```python
from build123d import *

# Parameters (mm, degrees)
SKETCH_1_W          = 43
SKETCH_1_H          = 21
EXTRUDE_1_DEPTH     = 1.6
SKETCH_2_R          = 1.5
CUT_EXTRUDE_1_DEPTH = 24.98040867
SKETCH_2_3_R        = 4
EXTRUDE_2_DEPTH     = 10.8
SKETCH_2_4_W        = 12
SKETCH_2_4_H        = 12
EXTRUDE_3_DEPTH     = 7.4
SKETCH_2_5_W        = 10
SKETCH_2_5_H        = 13
EXTRUDE_4_DEPTH     = 4.7
SKETCH_2_6_W        = 9
SKETCH_2_6_H        = 5
EXTRUDE_5_DEPTH     = 10
SKETCH_3_R          = 1.15
EXTRUDE_6_DEPTH     = 1.5


with BuildPart() as part:
    # Sketch 1 → Extrude 1 (new body)
    with BuildSketch(Plane(origin=(0, 0, 0), x_dir=(1, 0, 0), z_dir=(0, 1, 0))):
        Rectangle(SKETCH_1_W, SKETCH_1_H)
    extrude(amount=EXTRUDE_1_DEPTH)

    # Sketch 2 → Cut-Extrude 1 (cut, through all)
    with BuildSketch(Plane(origin=(0, 1.6, 0), x_dir=(1, 0, 0), z_dir=(0, 1, 0))):
        with Locations(Location((-15, 8, 0), (0, 0, 270))):
            Circle(SKETCH_2_R)
        with Locations(Location((15, -8, 0), (0, 0, 270))):
            Circle(SKETCH_2_R)
    extrude(amount=-CUT_EXTRUDE_1_DEPTH, mode=Mode.SUBTRACT)

    # Sketch 2_3 → Extrude 2 (add)
    with BuildSketch(Plane(origin=(0, 1.6, 0), x_dir=(1, 0, 0), z_dir=(0, 1, 0))):
        with Locations(Location((-17.5, 0, 0), (0, 0, 180))):
            Circle(SKETCH_2_3_R)
        with Locations((17.5, 0)):
            Circle(SKETCH_2_3_R)
    extrude(amount=EXTRUDE_2_DEPTH)

    # Sketch 2_4 → Extrude 3 (add)
    with BuildSketch(Plane(origin=(0, 1.6, 0), x_dir=(1, 0, 0), z_dir=(0, 1, 0))):
        with Locations((-5.5, -4.5)):
            Rectangle(SKETCH_2_4_W, SKETCH_2_4_H)
    extrude(amount=EXTRUDE_3_DEPTH)

    # Sketch 2_5 → Extrude 4 (add)
    with BuildSketch(Plane(origin=(0, 1.6, 0), x_dir=(1, 0, 0), z_dir=(0, 1, 0))):
        with Locations((6.5, -4)):
            Rectangle(SKETCH_2_5_W, SKETCH_2_5_H)
    extrude(amount=EXTRUDE_4_DEPTH)

    # Sketch 2_6 → Extrude 5 (add)
    with BuildSketch(Plane(origin=(0, 1.6, 0), x_dir=(1, 0, 0), z_dir=(0, 1, 0))):
        with Locations((-7, 7)):
            Rectangle(SKETCH_2_6_W, SKETCH_2_6_H)
    extrude(amount=EXTRUDE_5_DEPTH)

    # Sketch 3 → Extrude 6 (add)
    with BuildSketch(Plane(origin=(0, 11.6, 0), x_dir=(1, 0, 0), z_dir=(0, 1, 0))):
        with Locations(Location((-10.35, 8.35, 0), (0, 0, 90))):
            Circle(SKETCH_3_R)
    extrude(amount=EXTRUDE_6_DEPTH)


solid = part.part
```
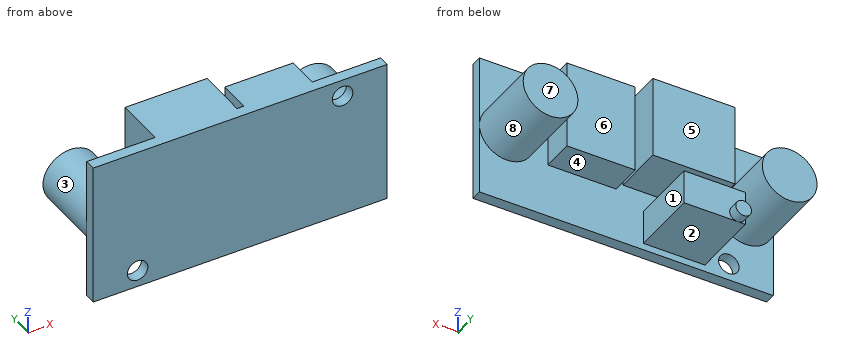
CAD build for the part. Positions are in the model's coordinates, mm. Face numbers are marked on the shaded views. A direction names the side the tool comes from. Round coordinates to 2 decimals unless told otherwise and drop trailing zeros. Loops run counter-clockwise (first coordinate to the right, second up) from the corner with the lowest first, then second, coordinate; pieces in that order, holes last. Notation, with made-up numbers: M 24,-9 L 73,-9 A19 cw 73,23 Z; hole C 52,43.5 d7. An arc over 180 degrees is marked long. Return JSON: item names as keys, results as strings. Group by question number.
(1) Saw through at D-D, the plane z = 5.75. List the corners of the cut face in (x, y), and give its area (3 significant figures).
(2) Tool access for the marked faces 4, 5, 6, 7 and 8: list every direction of +Z, -Z, +X, -X, +Y, -Y with a clear straight run to the whole face (end or side of a thin tool).
(3) Saw through at A-A, the plane z = 8. List the corners of the cut face in (x, y), and give its area (3 significant figures).
(4) Wall check: probe 1 along Z at (x, y) = (-10, 7); probe 2 along X at (y, z) = (4.5, 2.75); probe 3 along X at (y, z) = (0.3, 8). Give the ranges that are in metal, low to high. Write a range as [from, to].
(5) Saw through at C-C, the plane x = -15. List the corners of the cut face in (y, z), and give its area (3 significant figures).
(6) Drop flat-ended pins along their axis: P1, Ø2, axis at x = -2, z = 6.5, coming from the +Y side; P2, Ø5, axis at x = 15, z = 8, coming from the +Y side; P3, Ø4, axis at x = -16, z = -1.5, coming from the +Y side. Give the stop position or say it passes through.
(7) Saw through at B-B, the plane y = 5.75. List the corners of the cut face in (x, z).
(8) Mould opens along X. For the marked faces 1, 2 and 3 say: +X half, -X half, draft (parallel to the pull), parting line (faces both ways), or undercut.
Answer list:
{
 "1": {"outline": "M -21.5,0 L 21.5,0 L 21.5,1.6 L 11.5,1.6 L 11.5,6.3 L 1.5,6.3 L 1.5,1.6 L 0.5,1.6 L 0.5,9 L -11.5,9 L -11.5,1.6 L -21.5,1.6 Z", "area": "205 mm2"},
 "2": {"face 4": "-Z, +Y", "face 5": "+Z, +Y", "face 6": "+Z, -Z, +Y", "face 7": "+Z, -Z, +X, -X, +Y", "face 8": "+Y"},
 "3": {"outline": "M -21.5,0 L 13.5,0 L 13.5,1.6 L 11.5,1.6 L 11.5,6.3 L 1.5,6.3 L 1.5,1.6 L 0.5,1.6 L 0.5,9 L -11.5,9 L -11.5,1.6 L -21.5,1.6 Z; M 16.5,0 L 21.5,0 L 21.5,1.6 L 16.5,1.6 Z", "area": "200 mm2"},
 "4": {"probe 1": "[-9.5, -4.5], [-1.5, 10.5]", "probe 2": "[-20.4, -14.6], [-11.5, 0.5], [1.5, 11.5], [14.6, 20.4]", "probe 3": "[-21.5, 13.5], [16.5, 21.5]"},
 "5": {"outline": "M 0,-10.5 L 1.6,-10.5 L 1.6,-9.5 L 0,-9.5 Z; M 0,-6.5 L 1.6,-6.5 L 1.6,-3.12 L 12.4,-3.12 L 12.4,3.12 L 1.6,3.12 L 1.6,10.5 L 0,10.5 Z", "area": "96.2 mm2"},
 "6": {"P1": "y = 9", "P2": "y = 1.6", "P3": "y = 12.4"},
 "7": {"outline": "C -17.5,0 d8; M -11.5,-9.5 L -2.5,-9.5 L -2.5,-4.5 L -11.5,-4.5 Z; M -11.5,-1.5 L 0.5,-1.5 L 0.5,10.5 L -11.5,10.5 Z; M 1.5,-2.5 L 11.5,-2.5 L 11.5,10.5 L 1.5,10.5 Z; C 17.5,0 d8"},
 "8": {"face 1": "+X half", "face 2": "draft", "face 3": "undercut"}
}
